The model under review builds one solid part; all positions refer to its coordinate system, in mm. A direction names the side the tool comes from. Round coordinates to 2 decimals unless told otherwise and drop trailing zeros. Loops run counter-clockwise (first coordinate to the right, second up) from the corner with the lowest first, then second, coordinate; pieces in that order, holes last. Notation, with made-up numbers: M 33.5,-25.75 L 53.5,-25.75 A11 cw 53.5,-17.75 Z; hole C -30.75,43 d9. An arc over 180 degrees is marked long. Return JSON: item names as keys, results as strings. Group by question number.
Q1. For faces 1 (the face through (-250, 58, 40)), 2 (the face through (-123.25, 58.573, 35.972)), 3 (the face through (-123.25, 150.596, 60.428)), list the 3-axis set-ups (+Z, -Z, +X, -X, +Y, -Y) from which the entire face can be reached by the end or side of a thin tool; tool diameter is ignored.
Q2. Consider section B-B (y = 122). State the section outline as (x, z) points.
Q3. Clearance check with flat-ended pins moving along their axes: pin 1 Ø6 at (x, y) = (-109.5, 166) entering from -Z; pin 2 Ø2 at (x, y) = (-192, 103) entering from -Z; pin 3 Ø1 at (x, y) = (-93, -61) entering from +Z. State where each tip first meets the part, or that it passes through.
Q4. To check wall thickness, follow line 1 along Y through (x, z) = (-154, 6); line 2 along Z through (x, y) = (-15, 165); line 3 along Y through (x, z) = (-203.5, 23). State the ranges of each line that lie inside material, in increasing order.
Q5. Consider section C-C (y = -4.5). State the section outline as (x, z) points.
Q6. Draft analysis for pull direction Y (two halves, no side actions). For faces 4 (the face through (-123, 184.787, 35)), 5 (the face through (-123.25, 35.034, 31.178)), 6 (the face through (-123.25, 147.96, 59.84)), 7 (the face through (-123, -67.213, 13)), state which applies: pulls with the +Y half, pulls with the -Y half, needs draft (parallel to the pull), parting line crosses it, or undercut.
Q7. Consider section A-A (z = 44). State the section outline as (x, y) points.
from build123d import *

# Parameters (mm, degrees)
F1_DEPTH = 250


with BuildPart() as f1:
    # F0 (on Right) → F1 (new body)
    with BuildSketch(Plane.YZ):
        with BuildLine():
            Line((-67.213031, 23), (-67.213031, 3))
            ThreePointArc((-67.213031, 3), (-66.334352, 0.87868), (-64.213031, 0))
            Line((-64.213031, 0), (-64.213031, 1))
            Line((-64.213031, 1), (-59.013031, 1))
            Line((-59.013031, 1), (-59.013031, 0))
            Line((-59.013031, 0), (-57.193299, 0))
            Line((-57.193299, 0), (-57.193299, 1))
            Line((-57.193299, 1), (-49.393299, 1))
            ThreePointArc((-49.393299, 1), (-49.251877, 1.058579), (-49.193299, 1.2))
            Line((-49.193299, 1.2), (-49.193299, 3.8))
            ThreePointArc((-49.193299, 3.8), (-49.251877, 3.941421), (-49.393299, 4))
            Line((-49.393299, 4), (-63.213031, 4))
            ThreePointArc((-63.213031, 4), (-63.920138, 4.292893), (-64.213031, 5))
            Line((-64.213031, 5), (-64.213031, 23))
            ThreePointArc((-64.213031, 23), (-63.920138, 23.707107), (-63.213031, 24))
            Line((-63.213031, 24), (-60.213031, 24))
            ThreePointArc((-60.213031, 24), (-58.414842, 24.05394), (-56.623119, 24.215566))
            Line((-56.623119, 24.215566), (-54.620346, 24.456959))
            Line((-54.620346, 24.456959), (-51.939747, 24.780052))
            Line((-51.939747, 24.780052), (-49.457711, 25.079211))
            Line((-49.457711, 25.079211), (-46.777112, 25.402303))
            Line((-46.777112, 25.402303), (31.867868, 34.881367))
            Line((31.867868, 34.881367), (34.548467, 35.204459))
            Line((34.548467, 35.204459), (37.030503, 35.503618))
            Line((37.030503, 35.503618), (39.711102, 35.82671))
            Line((39.711102, 35.82671), (42.658329, 36.181939))
            ThreePointArc((42.658329, 36.181939), (45.213023, 36.581626), (47.733225, 37.160242))
            Line((47.733225, 37.160242), (52.531631, 38.441465))
            Line((52.531631, 38.441465), (55.140242, 39.13799))
            Line((55.140242, 39.13799), (57.555623, 39.782921))
            Line((57.555623, 39.782921), (60.164234, 40.479447))
            Line((60.164234, 40.479447), (141.917559, 62.308406))
            Line((141.917559, 62.308406), (144.52617, 63.004931))
            Line((144.52617, 63.004931), (146.941551, 63.649862))
            Line((146.941551, 63.649862), (149.550162, 64.346387))
            Line((149.550162, 64.346387), (156.589742, 66.226026))
            Line((156.589742, 66.226026), (180.786126, 66.246425))
            ThreePointArc((180.786126, 66.246425), (181.493777, 65.953831), (181.786969, 65.246426))
            Line((181.786969, 65.246426), (181.786969, 5))
            ThreePointArc((181.786969, 5), (181.494075, 4.292893), (180.786969, 4))
            Line((180.786969, 4), (162.786969, 4))
            ThreePointArc((162.786969, 4), (162.645547, 3.941421), (162.586969, 3.8))
            Line((162.586969, 3.8), (162.586969, 1.2))
            ThreePointArc((162.586969, 1.2), (162.645547, 1.058579), (162.786969, 1))
            Line((162.786969, 1), (170.586969, 1))
            Line((170.586969, 1), (170.586969, 0))
            Line((170.586969, 0), (174.586969, 0))
            Line((174.586969, 0), (174.586969, 1))
            Line((174.586969, 1), (179.786969, 1))
            Line((179.786969, 1), (179.786969, 0))
            ThreePointArc((179.786969, 0), (183.322503, 1.464466), (184.786969, 5))
            Line((184.786969, 5), (184.786969, 65.245583))
            ThreePointArc((184.786969, 65.245583), (183.321012, 68.782607), (179.782753, 70.245581))
            Line((179.782753, 70.245581), (160.415484, 70.229253))
            ThreePointArc((160.415484, 70.229253), (156.692023, 69.994123), (153.02654, 69.298648))
            Line((153.02654, 69.298648), (143.316564, 66.822088))
            Line((143.316564, 66.822088), (46.701335, 41.024851))
            ThreePointArc((46.701335, 41.024851), (44.45587, 40.509313), (42.179674, 40.153197))
            Line((42.179674, 40.153197), (-57.101774, 28.186824))
            ThreePointArc((-57.101774, 28.186824), (-58.654601, 28.046748), (-60.213031, 28))
            Line((-60.213031, 28), (-62.213031, 28))
            ThreePointArc((-62.213031, 28), (-65.748565, 26.535534), (-67.213031, 23))
        make_face()
        Polygon((-51.939747, 24.780052), (-54.620346, 24.456959), (-53.663036, 16.514444), (-50.982437, 16.837536), align=None)
        Polygon((-46.777112, 25.402303), (-49.457711, 25.079211), (-48.500401, 17.136695), (-45.819802, 17.459787), align=None)
        Polygon((34.548467, 35.204459), (31.867868, 34.881367), (32.825178, 26.938851), (35.505777, 27.261943), align=None)
        Polygon((39.711102, 35.82671), (37.030503, 35.503618), (37.987813, 27.561102), (40.668412, 27.884194), align=None)
        Polygon((55.140242, 39.13799), (52.531631, 38.441465), (54.59541, 30.712247), (57.204021, 31.408772), align=None)
        Polygon((151.613941, 56.617169), (149.550162, 64.346387), (146.941551, 63.649862), (149.00533, 55.920644), align=None)
        Polygon((60.164234, 40.479447), (57.555623, 39.782921), (59.619402, 32.053703), (62.228013, 32.750228), align=None)
        Polygon((146.589949, 55.275713), (144.52617, 63.004931), (141.917559, 62.308406), (143.981338, 54.579187), align=None)
    extrude(amount=-F1_DEPTH)


solid = f1.part
Values:
{
 "1": {"face 1": "+Z, -Z, -X, +Y, -Y", "face 2": "-Z, +X, -X", "face 3": "+X, -X"},
 "2": {"outline": "M -250,56.99 L 0,56.99 L 0,61.13 L -250,61.13 Z"},
 "3": {"pin 1": "stops at z = 1", "pin 2": "stops at z = 51.65", "pin 3": "stops at z = 28"},
 "4": {"line 1": "y = -67.21 to -64.21, 181.79 to 184.79", "line 2": "z = 1 to 4, 66.23 to 70.23", "line 3": "y = -67.21 to -64.21, -54.44 to -51.73, -49.21 to -46.49, 181.79 to 184.79"},
 "5": {"outline": "M -250,30.5 L 0,30.5 L 0,34.53 L -250,34.53 Z"},
 "6": {"face 4": "pulls with the +Y half", "face 5": "undercut", "face 6": "undercut", "face 7": "pulls with the -Y half"},
 "7": {"outline": "M -250,57.84 L 0,57.84 L 0,73.35 L -250,73.35 Z; M -250,181.79 L 0,181.79 L 0,184.79 L -250,184.79 Z"}
}
